Check sheet for the modelled part. Datum: model origin and axes. Units: mm. Face numbers are marked on the shaded views. A direction names the side the tool comes from. Give positions to 0.01 mm unless a question says otherwise; leave off trailing zeros. Order: outer loops, then holes, each group sorted by start corner. A loop starts at its lowest first (then second) coordinate and runs counter-clockwise, first axis right, second up. Notation, with made-up numbers: (-31.5, -25.75) -> (13.5, -25.75) arc R7 ccw to (13.5, -16.75) -> close; hole circle Ø5 at (20.25, 61). An arc over 180 degrees is marked (long way). Answer in a Markdown table with one row per item. Add a question column.
(1) Cross-section at C-C (z = 92). Record the cut outline in (x, y).
(2) Cross-section at D-D (x = -54.5). Record the cut outline in (y, z), then the cut area to 3 significant figures.
(3) Release check for a two-part mould opening along Z. For the marked faces 1, 2 and 3 record: released by +Z, released by -Z, zero draft, split by the parting line, or undercut.
(4) Thickness scan on L1, parallel to Z at x = -7, y = 71; L2, parallel to X at y = 48, z = 92; L3, parallel to Y at x = -56, z = -81. Record the ranges inside material, lowest first. Write a range as [from, to].
(5) Cross-section at B-B (x = -2). Record the cut outline in (y, z), then the cut area to 3 significant figures.
(6) Go/stop test with flat-tipped pins: pin 1 (2.5 mm diameter, centred on x = -58.86, z = 97.94, fed in from -Y); pin 2 (1.5 mm diameter, centred on x = 56.5, z = 25.5, fed in from +Y). Record where each tip stops, or that it passes through.
(7) Cross-section at A-A (y = 60). Record the cut outline in (x, z), then the cut area to 3 significant figures.
(8) Set-up check for the marked faces 4 and 5: record each of +Z, -Z, +X, -X, +Y, -Y from which the full face is reachable in a straight line by a thin tool's end or side.
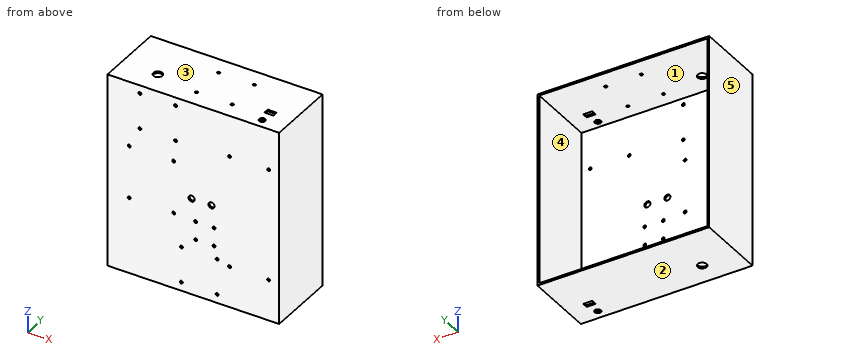
```python
from build123d import *

# Parameters (mm, degrees)
SKETCH2_W               = 189
SKETCH2_H               = 214
SKETCH2_W_2             = 185
SKETCH2_H_2             = 210
WALLS_DEPTH             = 75
SKETCH3_W               = 189
SKETCH3_H               = 214
BASE_DEPTH              = 2
SKETCH4_R               = 5
SKETCH4_W               = 10
SKETCH4_H               = 6
CUT_EXTRUDE1_DEPTH      = 246.66491406
SKETCH5_R               = 3.3782
CUT_EXTRUDE2_DEPTH      = 246.66491406
F_1_4_CLEARANCE_HOLE1_D = 6.7564
CUT_EXTRUDE3_REACH      = 164.198
SKETCH9_R               = 1.6
CUT_EXTRUDE4_REACH      = 247.665
SKETCH10_R              = 1.6


with BuildPart() as part:
    # Sketch2 → Walls (new body)
    with BuildSketch(Plane(origin=(0, 0, 0), x_dir=(1, 0, 0), z_dir=(0, 1, 0))):
        Rectangle(SKETCH2_W, SKETCH2_H)
        Rectangle(SKETCH2_W_2, SKETCH2_H_2, mode=Mode.SUBTRACT)
    extrude(amount=WALLS_DEPTH)

    # Sketch3 → Base (add)
    with BuildSketch(Plane.XZ):
        Rectangle(SKETCH3_W, SKETCH3_H)
    extrude(amount=BASE_DEPTH)

    # Sketch4 → Cut-Extrude1 (cut, through all)
    with BuildSketch(Plane(origin=(0, 0, -107), x_dir=(-1, 0, 0), z_dir=(0, 0, -1))):
        with Locations((54.5, 23)):
            Circle(SKETCH4_R)
        with Locations((-69.5, 23)):
            Rectangle(SKETCH4_W, SKETCH4_H)
    extrude(amount=-CUT_EXTRUDE1_DEPTH, mode=Mode.SUBTRACT)

    # Sketch5 → Cut-Extrude2 (cut, through all)
    with BuildSketch(Plane(origin=(0, 0, -107), x_dir=(-1, 0, 0), z_dir=(0, 0, -1))):
        with Locations((-69.5, 8.09625)):
            Circle(SKETCH5_R)
    extrude(amount=-CUT_EXTRUDE2_DEPTH, mode=Mode.SUBTRACT)

    # 1/4 Clearance Hole1 (through all)
    with Locations(Plane(origin=(0, -2, 0), x_dir=(-1, 0, 0), z_dir=(0, -1, 0))):
        with Locations((-20, 0), (2, 0)):
            Hole(F_1_4_CLEARANCE_HOLE1_D / 2)

    # Sketch9 → Cut-Extrude3 (cut, up to next)
    with BuildSketch(Plane.XZ.offset(2), mode=Mode.PRIVATE) as cut_extrude3_sk1:
        with Locations(Location((82.9, 61.675, 0), (0, 0, 270))):
            Circle(SKETCH9_R)
    cut_extrude3_tool1 = extrude(cut_extrude3_sk1.sketch, amount=-CUT_EXTRUDE3_REACH, mode=Mode.PRIVATE) & part.part
    # Sketch9 → Cut-Extrude3 (cut, up to next)
    with BuildSketch(Plane.XZ.offset(2), mode=Mode.PRIVATE) as cut_extrude3_sk2:
        with Locations(Location((82.9, -61.675, 0), (0, 0, 270))):
            Circle(SKETCH9_R)
    cut_extrude3_tool2 = extrude(cut_extrude3_sk2.sketch, amount=-CUT_EXTRUDE3_REACH, mode=Mode.PRIVATE) & part.part
    # Sketch9 → Cut-Extrude3 (cut, up to next)
    with BuildSketch(Plane.XZ.offset(2), mode=Mode.PRIVATE) as cut_extrude3_sk3:
        with Locations(Location((39.9, 61.675, 0), (0, 0, 270))):
            Circle(SKETCH9_R)
    cut_extrude3_tool3 = extrude(cut_extrude3_sk3.sketch, amount=-CUT_EXTRUDE3_REACH, mode=Mode.PRIVATE) & part.part
    # Sketch9 → Cut-Extrude3 (cut, up to next)
    with BuildSketch(Plane.XZ.offset(2), mode=Mode.PRIVATE) as cut_extrude3_sk4:
        with Locations(Location((39.9, -61.675, 0), (0, 0, 270))):
            Circle(SKETCH9_R)
    cut_extrude3_tool4 = extrude(cut_extrude3_sk4.sketch, amount=-CUT_EXTRUDE3_REACH, mode=Mode.PRIVATE) & part.part
    # Sketch9 → Cut-Extrude3 (cut, up to next)
    with BuildSketch(Plane.XZ.offset(2), mode=Mode.PRIVATE) as cut_extrude3_sk5:
        with Locations(Location((26.170769447, -58.141754017, 0), (0, 0, 270))):
            Circle(SKETCH9_R)
    cut_extrude3_tool5 = extrude(cut_extrude3_sk5.sketch, amount=-CUT_EXTRUDE3_REACH, mode=Mode.PRIVATE) & part.part
    # Sketch9 → Cut-Extrude3 (cut, up to next)
    with BuildSketch(Plane.XZ.offset(2), mode=Mode.PRIVATE) as cut_extrude3_sk6:
        with Locations(Location((26.170769447, -97.441754017, 0), (0, 0, 270))):
            Circle(SKETCH9_R)
    cut_extrude3_tool6 = extrude(cut_extrude3_sk6.sketch, amount=-CUT_EXTRUDE3_REACH, mode=Mode.PRIVATE) & part.part
    # Sketch9 → Cut-Extrude3 (cut, up to next)
    with BuildSketch(Plane.XZ.offset(2), mode=Mode.PRIVATE) as cut_extrude3_sk7:
        with Locations(Location((-13.129230553, -58.141754017, 0), (0, 0, 270))):
            Circle(SKETCH9_R)
    cut_extrude3_tool7 = extrude(cut_extrude3_sk7.sketch, amount=-CUT_EXTRUDE3_REACH, mode=Mode.PRIVATE) & part.part
    # Sketch9 → Cut-Extrude3 (cut, up to next)
    with BuildSketch(Plane.XZ.offset(2), mode=Mode.PRIVATE) as cut_extrude3_sk8:
        with Locations(Location((-13.129230553, -97.441754017, 0), (0, 0, 270))):
            Circle(SKETCH9_R)
    cut_extrude3_tool8 = extrude(cut_extrude3_sk8.sketch, amount=-CUT_EXTRUDE3_REACH, mode=Mode.PRIVATE) & part.part
    # Sketch9 → Cut-Extrude3 (cut, up to next)
    with BuildSketch(Plane.XZ.offset(2), mode=Mode.PRIVATE) as cut_extrude3_sk9:
        with Locations(Location((22.84154278, -24.185222858, 0), (0, 0, 270))):
            Circle(SKETCH9_R)
    cut_extrude3_tool9 = extrude(cut_extrude3_sk9.sketch, amount=-CUT_EXTRUDE3_REACH, mode=Mode.PRIVATE) & part.part
    # Sketch9 → Cut-Extrude3 (cut, up to next)
    with BuildSketch(Plane.XZ.offset(2), mode=Mode.PRIVATE) as cut_extrude3_sk10:
        with Locations(Location((22.84154278, -44.485222858, 0), (0, 0, 270))):
            Circle(SKETCH9_R)
    cut_extrude3_tool10 = extrude(cut_extrude3_sk10.sketch, amount=-CUT_EXTRUDE3_REACH, mode=Mode.PRIVATE) & part.part
    # Sketch9 → Cut-Extrude3 (cut, up to next)
    with BuildSketch(Plane.XZ.offset(2), mode=Mode.PRIVATE) as cut_extrude3_sk11:
        with Locations(Location((2.54154278, -24.185222858, 0), (0, 0, 270))):
            Circle(SKETCH9_R)
    cut_extrude3_tool11 = extrude(cut_extrude3_sk11.sketch, amount=-CUT_EXTRUDE3_REACH, mode=Mode.PRIVATE) & part.part
    # Sketch9 → Cut-Extrude3 (cut, up to next)
    with BuildSketch(Plane.XZ.offset(2), mode=Mode.PRIVATE) as cut_extrude3_sk12:
        with Locations(Location((2.54154278, -44.485222858, 0), (0, 0, 270))):
            Circle(SKETCH9_R)
    cut_extrude3_tool12 = extrude(cut_extrude3_sk12.sketch, amount=-CUT_EXTRUDE3_REACH, mode=Mode.PRIVATE) & part.part
    # Sketch9 → Cut-Extrude3 (cut, up to next)
    with BuildSketch(Plane.XZ.offset(2), mode=Mode.PRIVATE) as cut_extrude3_sk13:
        with Locations(Location((-21.583449299, 35.175065187, 0), (0, 0, 270))):
            Circle(SKETCH9_R)
    cut_extrude3_tool13 = extrude(cut_extrude3_sk13.sketch, amount=-CUT_EXTRUDE3_REACH, mode=Mode.PRIVATE) & part.part
    # Sketch9 → Cut-Extrude3 (cut, up to next)
    with BuildSketch(Plane.XZ.offset(2), mode=Mode.PRIVATE) as cut_extrude3_sk14:
        with Locations(Location((-21.583449299, -22.824934813, 0), (0, 0, 270))):
            Circle(SKETCH9_R)
    cut_extrude3_tool14 = extrude(cut_extrude3_sk14.sketch, amount=-CUT_EXTRUDE3_REACH, mode=Mode.PRIVATE) & part.part
    # Sketch9 → Cut-Extrude3 (cut, up to next)
    with BuildSketch(Plane.XZ.offset(2), mode=Mode.PRIVATE) as cut_extrude3_sk15:
        with Locations(Location((-70.583449299, -22.824934813, 0), (0, 0, 270))):
            Circle(SKETCH9_R)
    cut_extrude3_tool15 = extrude(cut_extrude3_sk15.sketch, amount=-CUT_EXTRUDE3_REACH, mode=Mode.PRIVATE) & part.part
    # Sketch9 → Cut-Extrude3 (cut, up to next)
    with BuildSketch(Plane.XZ.offset(2), mode=Mode.PRIVATE) as cut_extrude3_sk16:
        with Locations(Location((-70.583449299, 35.175065187, 0), (0, 0, 270))):
            Circle(SKETCH9_R)
    cut_extrude3_tool16 = extrude(cut_extrude3_sk16.sketch, amount=-CUT_EXTRUDE3_REACH, mode=Mode.PRIVATE) & part.part
    # Sketch9 → Cut-Extrude3 (cut, up to next)
    with BuildSketch(Plane.XZ.offset(2), mode=Mode.PRIVATE) as cut_extrude3_sk17:
        with Locations(Location((-58.856871361, 58.63750142, 0), (0, 0, 270))):
            Circle(SKETCH9_R)
    cut_extrude3_tool17 = extrude(cut_extrude3_sk17.sketch, amount=-CUT_EXTRUDE3_REACH, mode=Mode.PRIVATE) & part.part
    # Sketch9 → Cut-Extrude3 (cut, up to next)
    with BuildSketch(Plane.XZ.offset(2), mode=Mode.PRIVATE) as cut_extrude3_sk18:
        with Locations(Location((-19.556871361, 58.63750142, 0), (0, 0, 270))):
            Circle(SKETCH9_R)
    cut_extrude3_tool18 = extrude(cut_extrude3_sk18.sketch, amount=-CUT_EXTRUDE3_REACH, mode=Mode.PRIVATE) & part.part
    # Sketch9 → Cut-Extrude3 (cut, up to next)
    with BuildSketch(Plane.XZ.offset(2), mode=Mode.PRIVATE) as cut_extrude3_sk19:
        with Locations(Location((-19.556871361, 97.93750142, 0), (0, 0, 270))):
            Circle(SKETCH9_R)
    cut_extrude3_tool19 = extrude(cut_extrude3_sk19.sketch, amount=-CUT_EXTRUDE3_REACH, mode=Mode.PRIVATE) & part.part
    # Sketch9 → Cut-Extrude3 (cut, up to next)
    with BuildSketch(Plane.XZ.offset(2), mode=Mode.PRIVATE) as cut_extrude3_sk20:
        with Locations(Location((-58.856871361, 97.93750142, 0), (0, 0, 270))):
            Circle(SKETCH9_R)
    cut_extrude3_tool20 = extrude(cut_extrude3_sk20.sketch, amount=-CUT_EXTRUDE3_REACH, mode=Mode.PRIVATE) & part.part
    add(cut_extrude3_tool1.solids().sort_by_distance((82.9, -2, 61.675))[0], mode=Mode.SUBTRACT)
    add(cut_extrude3_tool2.solids().sort_by_distance((82.9, -2, -61.675))[0], mode=Mode.SUBTRACT)
    add(cut_extrude3_tool3.solids().sort_by_distance((39.9, -2, 61.675))[0], mode=Mode.SUBTRACT)
    add(cut_extrude3_tool4.solids().sort_by_distance((39.9, -2, -61.675))[0], mode=Mode.SUBTRACT)
    add(cut_extrude3_tool5.solids().sort_by_distance((26.170769, -2, -58.141754))[0], mode=Mode.SUBTRACT)
    add(cut_extrude3_tool6.solids().sort_by_distance((26.170769, -2, -97.441754))[0], mode=Mode.SUBTRACT)
    add(cut_extrude3_tool7.solids().sort_by_distance((-13.129231, -2, -58.141754))[0], mode=Mode.SUBTRACT)
    add(cut_extrude3_tool8.solids().sort_by_distance((-13.129231, -2, -97.441754))[0], mode=Mode.SUBTRACT)
    add(cut_extrude3_tool9.solids().sort_by_distance((22.841543, -2, -24.185223))[0], mode=Mode.SUBTRACT)
    add(cut_extrude3_tool10.solids().sort_by_distance((22.841543, -2, -44.485223))[0], mode=Mode.SUBTRACT)
    add(cut_extrude3_tool11.solids().sort_by_distance((2.541543, -2, -24.185223))[0], mode=Mode.SUBTRACT)
    add(cut_extrude3_tool12.solids().sort_by_distance((2.541543, -2, -44.485223))[0], mode=Mode.SUBTRACT)
    add(cut_extrude3_tool13.solids().sort_by_distance((-21.583449, -2, 35.175065))[0], mode=Mode.SUBTRACT)
    add(cut_extrude3_tool14.solids().sort_by_distance((-21.583449, -2, -22.824935))[0], mode=Mode.SUBTRACT)
    add(cut_extrude3_tool15.solids().sort_by_distance((-70.583449, -2, -22.824935))[0], mode=Mode.SUBTRACT)
    add(cut_extrude3_tool16.solids().sort_by_distance((-70.583449, -2, 35.175065))[0], mode=Mode.SUBTRACT)
    add(cut_extrude3_tool17.solids().sort_by_distance((-58.856871, -2, 58.637501))[0], mode=Mode.SUBTRACT)
    add(cut_extrude3_tool18.solids().sort_by_distance((-19.556871, -2, 58.637501))[0], mode=Mode.SUBTRACT)
    add(cut_extrude3_tool19.solids().sort_by_distance((-19.556871, -2, 97.937501))[0], mode=Mode.SUBTRACT)
    add(cut_extrude3_tool20.solids().sort_by_distance((-58.856871, -2, 97.937501))[0], mode=Mode.SUBTRACT)

    # Sketch10 → Cut-Extrude4 (cut, up to next)
    with BuildSketch(Plane.XY.offset(107), mode=Mode.PRIVATE) as cut_extrude4_sk1:
        with Locations((-7.650141085, 55.256030586)):
            Circle(SKETCH10_R)
    cut_extrude4_tool1 = extrude(cut_extrude4_sk1.sketch, amount=-CUT_EXTRUDE4_REACH, mode=Mode.PRIVATE) & part.part
    # Sketch10 → Cut-Extrude4 (cut, up to next)
    with BuildSketch(Plane.XY.offset(107), mode=Mode.PRIVATE) as cut_extrude4_sk2:
        with Locations((31.649858915, 55.256030586)):
            Circle(SKETCH10_R)
    cut_extrude4_tool2 = extrude(cut_extrude4_sk2.sketch, amount=-CUT_EXTRUDE4_REACH, mode=Mode.PRIVATE) & part.part
    # Sketch10 → Cut-Extrude4 (cut, up to next)
    with BuildSketch(Plane.XY.offset(107), mode=Mode.PRIVATE) as cut_extrude4_sk3:
        with Locations((31.649858915, 15.956030586)):
            Circle(SKETCH10_R)
    cut_extrude4_tool3 = extrude(cut_extrude4_sk3.sketch, amount=-CUT_EXTRUDE4_REACH, mode=Mode.PRIVATE) & part.part
    # Sketch10 → Cut-Extrude4 (cut, up to next)
    with BuildSketch(Plane.XY.offset(107), mode=Mode.PRIVATE) as cut_extrude4_sk4:
        with Locations((-7.650141085, 15.956030586)):
            Circle(SKETCH10_R)
    cut_extrude4_tool4 = extrude(cut_extrude4_sk4.sketch, amount=-CUT_EXTRUDE4_REACH, mode=Mode.PRIVATE) & part.part
    add(cut_extrude4_tool1.solids().sort_by_distance((-7.650141, 55.256031, 107))[0], mode=Mode.SUBTRACT)
    add(cut_extrude4_tool2.solids().sort_by_distance((31.649859, 55.256031, 107))[0], mode=Mode.SUBTRACT)
    add(cut_extrude4_tool3.solids().sort_by_distance((31.649859, 15.956031, 107))[0], mode=Mode.SUBTRACT)
    add(cut_extrude4_tool4.solids().sort_by_distance((-7.650141, 15.956031, 107))[0], mode=Mode.SUBTRACT)


solid = part.part
```
Answer below:
| question | item | result |
|---|---|---|
| 1 | outline | (-94.5, -2) -> (94.5, -2) -> (94.5, 75) -> (92.5, 75) -> (92.5, 0) -> (-92.5, 0) -> (-92.5, 75) -> (-94.5, 75) -> close |
| 2 | outline | (-2, -107) -> (18, -107) -> (18, -105) -> (0, -105) -> (0, 105) -> (18, 105) -> (18, 107) -> (-2, 107) -> close; (28, -107) -> (75, -107) -> (75, -105) -> (28, -105) -> close; (28, 105) -> (75, 105) -> (75, 107) -> (28, 107) -> close |
| 2 | area | 688 mm² |
| 3 | face 1 | undercut |
| 3 | face 2 | released by -Z |
| 3 | face 3 | released by +Z |
| 4 | L1 | z = [-107, -105], [105, 107] |
| 4 | L2 | x = [-94.5, -92.5], [92.5, 94.5] |
| 4 | L3 | y = [-2, 0] |
| 5 | outline | (-2, -107) -> (75, -107) -> (75, -105) -> (0, -105) -> (0, -3.38) -> (-2, -3.38) -> close; (-2, 3.38) -> (0, 3.38) -> (0, 105) -> (75, 105) -> (75, 107) -> (-2, 107) -> close |
| 5 | area | 714 mm² |
| 6 | pin 1 | passes through |
| 6 | pin 2 | stops at y = 0 |
| 7 | outline | (-94.5, -107) -> (94.5, -107) -> (94.5, 107) -> (-94.5, 107) -> close; hole (-92.5, -105) -> (92.5, -105) -> (92.5, 105) -> (-92.5, 105) -> close |
| 7 | area | 1,600 mm² |
| 8 | face 4 | +Y |
| 8 | face 5 | +Z, -Z, -X, +Y, -Y |
